Could you check a few things on this model? Use its own coordinates, in mm. Face numbers are marked on the shaded views. A direction names the side the tool comes from. Round coordinates to 2 decimals unless told otherwise and drop trailing zeros. Write each loop counter-clockwise with the first axis right and the second up, starting at its lowest first coordinate (ties: lowest second). Pieces come first, ordered by that corner, then holes. Notation, with made-up numbers: (10, -4.75) -> (27, -4.75) arc R25 ccw to (27, 15.25) -> close; hole circle Ø3 at (-29.5, 2). An arc over 180 degrees is marked (long way). One line per question, with ' | ' between items. Start each with the question number.
1. Imagine slicing it at C-C, the plane x = -1. List the corners of the cut face in (y, z) for me (3 decimals).
2. If I drill on line 1 along X through (y, z) = (4, 9.25); line 2 along Y through (x, z) = (29, 10.25) (3 decimals); line 3 along Y through (x, z) = (19, 8.25) (3 decimals), over which ranges is the centre line in solid material (lowest first)? Write a range as [from, to].
3. Imagine slicing it at D-D, the plane x = 35. List the corners of the cut face in (y, z) for me (3 decimals).
4. Thinking about a two-plate mould opening in Y: for the marked faces 1, 2 and 3, which applies, released by +Y, released by -Y, zero draft, split by the parting line, or undercut?
5. For the marked faces 4 and 5, which set-ups out of +Z, -Z, +X, -X, +Y, -Y let a thin tool reach every point of the face, with its end or its side?
6. Imagine slicing it at B-B, the plane y = 59.5. List the corners of the cut face in (x, z) for me (3 decimals), and give its area (3 significant figures).
7. Imagine slicing it at A-A, the plane z = 6.25. List the corners of the cut face in (x, y) for me (3 decimals).
8. For pin 1 Ø3 at (y, z) = (10, 7) entering from -X; pin 2 Ø10 at (x, y) = (-5, 13.5) entering from +Z (3 decimals); pin 3 Ø6 at (x, z) = (16, 7) entering from +Y; pin 4 Ø8 at (x, z) = (18, 8.5) entering from +Y, each with a flat end and sliding along its axis, tell me the tip position at first contact or that it passes through.
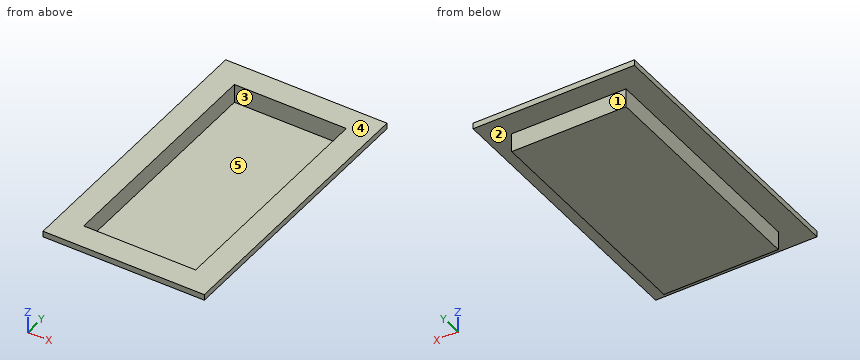
from build123d import *

# Parameters (mm, degrees)
F0_W     = 61.722
F0_H     = 127
F1_DEPTH = 10.16
F2_W     = 87.122
F2_H     = 152.4
F3_DEPTH = 3.175
F4_W     = 60.452
F4_H     = 125.73
F5_DEPTH = 10.16


with BuildPart() as f1:
    # F0 (on Top) → F1 (new body)
    with BuildSketch(Plane.XY):
        Rectangle(F0_W, F0_H)
    extrude(amount=F1_DEPTH)

    # F2 (on face) → F3 (join)
    with BuildSketch(Plane.XY.offset(10.16)):
        Rectangle(F2_W, F2_H)
    extrude(amount=F3_DEPTH)

    # F4 (on face) → F5 (cut)
    with BuildSketch(Plane.XY.offset(13.335)):
        Rectangle(F4_W, F4_H)
    extrude(amount=-F5_DEPTH, mode=Mode.SUBTRACT)


solid = f1.part
Geometry results:
1) outline: (-76.2, 10.16) -> (-63.5, 10.16) -> (-63.5, 0) -> (63.5, 0) -> (63.5, 10.16) -> (76.2, 10.16) -> (76.2, 13.335) -> (62.865, 13.335) -> (62.865, 3.175) -> (-62.865, 3.175) -> (-62.865, 13.335) -> (-76.2, 13.335) -> close
2) line 1: x = [-30.86, -30.23], [30.23, 30.86] | line 2: y = [-76.2, -62.865], [62.865, 76.2] | line 3: y = [-63.5, -62.865], [62.865, 63.5]
3) outline: (-76.2, 10.16) -> (76.2, 10.16) -> (76.2, 13.335) -> (-76.2, 13.335) -> close
4) face 1: released by +Y | face 2: zero draft | face 3: undercut
5) face 4: +Z, +X, -X, +Y, -Y | face 5: +Z
6) outline: (-43.561, 10.16) -> (-30.861, 10.16) -> (-30.861, 0) -> (30.861, 0) -> (30.861, 10.16) -> (43.561, 10.16) -> (43.561, 13.335) -> (30.226, 13.335) -> (30.226, 3.175) -> (-30.226, 3.175) -> (-30.226, 13.335) -> (-43.561, 13.335) -> close | area: 290 mm2
7) outline: (-30.861, -63.5) -> (30.861, -63.5) -> (30.861, 63.5) -> (-30.861, 63.5) -> close; hole (-30.226, -62.865) -> (30.226, -62.865) -> (30.226, 62.865) -> (-30.226, 62.865) -> close
8) pin 1: stops at x = -30.86 | pin 2: stops at z = 3.175 | pin 3: stops at y = 63.5 | pin 4: stops at y = 76.2
